Geometry: final body of the model. Coordinates: model frame, mm. A direction names the side the tool comes from. Coordinates: 2 decimals unless noted, no trailing zeros. Loops run counter-clockwise (first coordinate to the right, second up) from the corner with the lowest first, then second, coordinate; pieces in that order, holes last. Notation, with made-up numbers: M 28.25,9 L 59.25,9 A26 cw 59.25,41 Z; hole C 23,1 d10. An arc over 180 degrees is marked long. Write item = value, one per line. Start each with the question number.
```python
from build123d import *

# Parameters (mm, degrees)
SKETCH3_R                = 3.9
BOSS_EXTRUDE1_DEPTH      = 2
BOSS_EXTRUDE1_DEPTH_BACK = 2
SKETCH5_R                = 0.5
BOSS_EXTRUDE4_DEPTH      = 2
SKETCH4_R                = 2.25
CUT_EXTRUDE1_DEPTH       = 3


with BuildPart() as part:
    # Sketch3 → Boss-Extrude1 (new body, two sides)
    with BuildSketch(Plane(origin=(0, 0, 0), x_dir=(1, 0, 0), z_dir=(0, 1, 0))) as boss_extrude1_sk:
        with Locations((-5.706641347, -37.429153992)):
            Circle(SKETCH3_R)
    extrude(amount=BOSS_EXTRUDE1_DEPTH)
    extrude(boss_extrude1_sk.sketch, amount=-BOSS_EXTRUDE1_DEPTH_BACK)

    # Sketch5 → Boss-Extrude4 (add)
    with BuildSketch(Plane(origin=(0, 0, 0), x_dir=(1, 0, 0), z_dir=(0, 1, 0))):
        with BuildLine():
            Line((8.943358653, -35.679153992), (-5.706641347, -34.108983126))
            Line((-5.706641347, -34.108983126), (-20.356641347, -35.679153992))
            ThreePointArc((-20.356641347, -35.679153992), (-22.106641347, -37.429153992), (-20.356641347, -39.179153992))
            Line((-20.356641347, -39.179153992), (-5.706641347, -40.749324858))
            Line((-5.706641347, -40.749324858), (8.943358653, -39.179153992))
            ThreePointArc((8.943358653, -39.179153992), (10.693358653, -37.429153992), (8.943358653, -35.679153992))
        make_face()
        with Locations((8.943358653, -37.429153992)):
            Circle(SKETCH5_R, mode=Mode.SUBTRACT)
        with Locations((-20.356641347, -37.429153992)):
            Circle(SKETCH5_R, mode=Mode.SUBTRACT)
    extrude(amount=BOSS_EXTRUDE4_DEPTH)

    # Sketch4 → Cut-Extrude1 (cut, through all)
    with BuildSketch(Plane(origin=(0, 0, 0), x_dir=(1, 0, 0), z_dir=(0, 1, 0))):
        with Locations((-5.706641347, -37.429153992)):
            Circle(SKETCH4_R)
    extrude(amount=-CUT_EXTRUDE1_DEPTH, mode=Mode.SUBTRACT)


solid = part.part
```
Item 1: Line query: line 1 (X direction, y = 1.4, z = 37.5); line 2 (Y direction, x = 6, z = 37); line 3 (Z direction, x = -5.5, y = -0.45). Output: solid intervals per line, ascending. Write a range as from..to.
Item 2: First-contact query: pin 1 (4 mm diameter, centred on x = -17, z = 39.5, fed in from -Y). Flat tip, straight axial feed; report the tip coordinate or a pass-through.
Item 3: Reachability of faces 1 (the cylindrical face through (-2.104, -0.416, 38.923)), 2 (the flat face through (-14.154, 0.986, 35.014)) from +Z, -Z, +X, -X, +Y, -Y: full face, straight path, thin tool, end or side. Return the list, or none.
Item 4: Section query D-D (y = -0.85). Return the cut outline in (x, z).
Item 5: Section query A-A (y = 0.95). Return the cut outline in (x, z), plus the area to 3 significant figures.
Item 6: Pull-direction query (X, two-part tool) for faces 3 (the flat face through (-14.325, 0.986, 39.826)), 4 (the cylindrical face through (-6, -1, 35.2)), 5 (the flat face through (-6, -2, 40)); classes: released by +X, released by -X, zero draft, split by the parting line, or undercut.
Item 7: Section query C-C (x = -4). Return the cut outline in (y, z), plus the area to 3 significant figures.
Item 8: Section query B-B (z = 36.5). Return the cut outline in (x, y).
Verdict:
q1.line_1 = -22.11..-20.85, -19.86..8.45, 9.44..10.69
q1.line_2 = 0..2
q1.line_3 = 33.53..35.19, 39.67..41.32
q2.pin_1 = 0
q3.face_1 = -Y
q3.face_2 = -Z, -X, +Y, -Y
q4.outline = C -5.71,37.43 d7.8; hole C -5.71,37.43 d4.5
q5.outline = M -20.36,35.68 L -8.12,34.37 A3.9 ccw -3.29,34.37 L 8.94,35.68 A1.75 ccw 8.94,39.18 L -3.29,40.49 A3.9 ccw -8.12,40.49 L -20.36,39.18 A1.75 ccw Z; hole C -20.36,37.43 d1; hole C 8.94,37.43 d1
q5.area = 161 mm2
q6.face_3 = released by -X
q6.face_4 = undercut
q6.face_5 = zero draft
q7.outline = M -2,33.92 L 2,33.92 L 2,40.94 L -2,40.94 L -2,38.9 L 0,38.9 L 0,35.96 L -2,35.96 Z
q7.area = 22.2 mm2
q8.outline = M -21.84,0 L -9.49,0 L -9.49,-2 L -7.76,-2 L -7.76,0 L -3.66,0 L -3.66,-2 L -1.92,-2 L -1.92,0 L 10.43,0 L 10.43,2 L -21.84,2 Z
